from build123d import *

# Parameters (mm, degrees)
SKETCH1_W           = 20
SKETCH1_H           = 20
BOSS_EXTRUDE1_DEPTH = 20
CUT_EXTRUDE_X_DEPTH = 1
CUT_EXTRUDE_Y_DEPTH = 1
CUT_EXTRUDE_Z_DEPTH = 1


with BuildPart() as part:
    # Sketch1 → Boss-Extrude1 (new body)
    with BuildSketch(Plane.XY):
        Rectangle(SKETCH1_W, SKETCH1_H)
    extrude(amount=BOSS_EXTRUDE1_DEPTH)

    # Sketch2 → Cut-Extrude X (cut)
    with BuildSketch(Plane.XY.offset(20)):
        Polygon((-3.653846154, 5), (-2.618189103, 5), (0, 0.909455128), (2.618189103, 5), (3.653846154, 5), (0.518830128, 0.100160256), (3.782051282, -5), (2.746394231, -5), (0, -0.709134615), (-2.746394231, -5), (-3.782051282, -5), (-0.516826923, 0.100160256), align=None)
    extrude(amount=-CUT_EXTRUDE_X_DEPTH, mode=Mode.SUBTRACT)

    # Sketch3 → Cut-Extrude Y (cut)
    with BuildSketch(Plane(origin=(10, 0, 0), x_dir=(0, 0, -1), z_dir=(1, 0, 0))):
        Polygon((-13.653846154, 5), (-12.626201923, 5), (-9.997996795, 0.703125), (-7.373798077, 5), (-6.346153846, 5), (-9.551282051, -0.246394231), (-9.551282051, -5), (-10.448717949, -5), (-10.448717949, -0.246394231), align=None)
    extrude(amount=-CUT_EXTRUDE_Y_DEPTH, mode=Mode.SUBTRACT)

    # Sketch4 → Cut-Extrude Z (cut)
    with BuildSketch(Plane(origin=(0, 10, 0), x_dir=(1, 0, 0), z_dir=(0, 1, 0))):
        Polygon((-3.974358974, -7.435897436), (-5, -7.435897436), (-5, -12.692307692), (3.974358974, -8.497596154), (3.974358974, -12.564102564), (5, -12.564102564), (5, -7.051282051), (-3.974358974, -11.24599359), align=None)
    extrude(amount=-CUT_EXTRUDE_Z_DEPTH, mode=Mode.SUBTRACT)


solid = part.part
Design review of the part built by this model. Coordinates are the model's own, in mm. A direction names the side the tool comes from. Coordinates: 2 decimals unless noted, no trailing zeros.
Item 1: Wall thickness on L1, parallel to X at y = 9.25, z = 10.25; L2, parallel to Y at x = -3.25, z = 11.5: over which ranges is each line inside the solid? List them lowest first.
Completed:
L1: x = -10 to -5, -3.97 to -1.84, 0.23 to 3.97, 5 to 10
L2: y = -10 to 9
Item 2: For faces 5 (the flat face through (4.5, 9.5, 12.564)), 6 (the flat face through (-1.327, 2.983, 19.507)), 7 (the flat face through (9.5, -5, 10)), list the 3-axis set-ups (+Z, -Z, +X, -X, +Y, -Y) from which the entire face can be reached by the end or side of a thin tool; tool diameter is ignored.
Completed:
face 5: +Y
face 6: +Z
face 7: +X
Item 3: Draft analysis for pull direction Y (two halves, no side actions). For faces 1 (the flat face through (9.51, 2.41, 7.93)), 2 (the flat face through (1.4, -2.9, 19.5)), 3 (the flat face through (0, 10, 12)), 4 (the flat face through (2, 0, 20)), state which applies: pulls with the +Y half, pulls with the -Y half, needs draft (parallel to the pull), parting line crosses it, or undercut.
Completed:
face 1: undercut
face 2: undercut
face 3: pulls with the +Y half
face 4: needs draft
